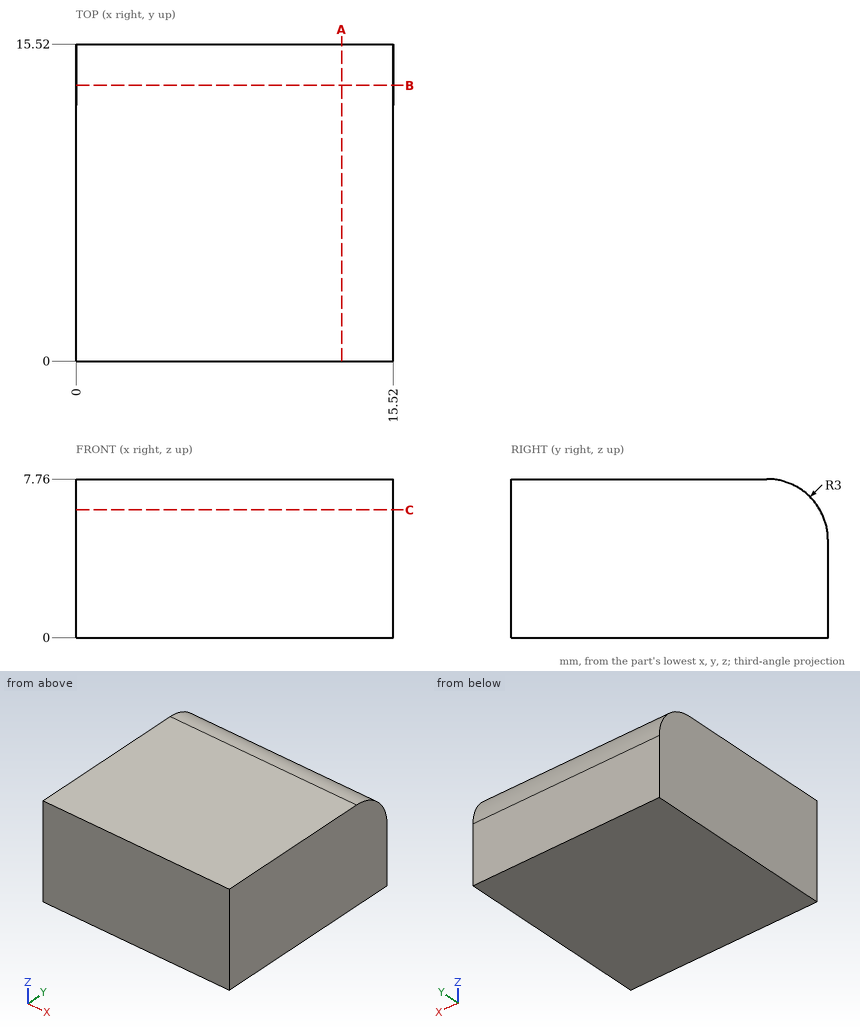
For this review, use the dimensioned drawing (mm, ordinates from the lowest corner) and the shaded views. Give positions to 0.01 mm unless a question says otherwise; leave off trailing zeros. Loops run counter-clockwise (first coordinate to the right, second up) from the corner with the lowest first, then second, coordinate; pieces in that order, holes last.
Item 1: For line 1 along Z through (x, y) = (11, 13.5); line 2 along Z through (x, y) = (12.75, 14.75); line 3 along Y through (x, z) = (13.25, 7.5), list the stretches that pass through material, from the lowest coordinate up.
Item 2: Insertion check: pin 1 (1.5 mm diameter, centred on x = 3, z = 7, fed in from +Y). The pin has a flat end and moves straight along its axis. Give the tip position at first contact, or say it passes through.
Item 3: Take a section at A-A, the plane x = 13. State the section outline as (y, z) points, and give its area (3 significant figures).
Item 4: Take a section at B-B, the plane y = 13.5. State the section outline as (x, z) points.
Item 5: Take a section at C-C, the plane z = 6.25. State the section outline as (x, y) points, and give its area (3 significant figures).
Calculated:
1. line 1: z = 0 to 7.6
1. line 2: z = 0 to 6.77
1. line 3: y = 0 to 13.74
2. pin 1: stops at y = 15.12
3. outline: (0, 0) - (15.52, 0) - (15.52, 4.76) arc R3 ccw to (12.52, 7.76) - (0, 7.76) - close
3. area: 119 mm2
4. outline: (0, 0) - (15.52, 0) - (15.52, 7.6) - (0, 7.6) - close
5. outline: (0, 0) - (15.52, 0) - (15.52, 15.12) - (0, 15.12) - close
5. area: 235 mm2
